from build123d import *

# Parameters (mm, degrees)
F0_W     = 20
F0_H     = 20
F1_DEPTH = 30
F3_D     = 8
F3_DEPTH = 50
F3_TIP   = 2.4034424761
F4_R     = 5
F5_W     = 20
F5_H     = 13
F6_DEPTH = 0.5


# Not quite as in the source:
# - a feature names something its author has since deleted; it is built from what else it names


with BuildPart() as f1:
    # F0 (on Right) → F1 (new body)
    with BuildSketch(Plane.YZ):
        with Locations((-10, 10)):
            Rectangle(F0_W, F0_H)
    extrude(amount=F1_DEPTH)

    # F3
    with Locations(Plane.YZ.offset(30)):
        with Locations((-10, 18.097827211)):
            Hole(F3_D / 2, depth=F3_DEPTH)
            with Locations((0, 0, -(F3_DEPTH + F3_TIP / 2))):  # 118° drill point
                Cone(0, F3_D / 2, F3_TIP, mode=Mode.SUBTRACT)

    # F4
    f4_edges = [f1.edges().sort_by_distance(p)[0] for p in [
        (30, -3.240615, 20),
        (30, -16.759385, 20),
        (15, -20, 20),
        (15, 0, 20),
        (0, -16.759385, 20),
        (0, -3.240615, 20),
    ]]
    fillet(f4_edges, radius=F4_R)

    # F5 (on face) → F6 (cut)
    with BuildSketch(Plane(origin=(0, 0, 0), x_dir=(1, 0, 0), z_dir=(0, 0, -1))):
        with Locations((15, 9.8333333333)):
            Rectangle(F5_W, F5_H)
    extrude(amount=-F6_DEPTH, mode=Mode.SUBTRACT)


solid = f1.part
Verification items for the finished model (mm, model axes). A direction names the side the tool comes from. Give positions to 0.01 mm unless a question says otherwise; leave off trailing zeros. Order: outer loops, then holes, each group sorted by start corner. A loop starts at its lowest first (then second) coordinate and runs counter-clockwise, first axis right, second up. Notation, with made-up numbers: M 60,6.5 L 66,6.5 A29 ccw 66,35.5 Z; hole C 50.25,49 d9. An arc over 180 degrees is marked long. Answer as a JSON object with one key per item and string values. Group by question number.
1) Mould release check, pull along Y, two halves, no side actions. Record for faces 1 (the face through (30, -10, 8)), 2 (the face through (14.8, -9.9, 14.1)), 3 (the face through (15, -2, 19)): released by +Y, released by -Y, zero draft, split by the parting line, or undercut.
2) Cross-section at C-C (x = 10.5). Enter the section's corners in (y, z).
3) Depth check by flat-ended pin: pin 1 Ø1.5 at (y, z) = (-15, 16.5) entering from -X; pin 2 Ø4 at (x, y) = (18.5, -9.5) entering from -Z. Enter the tip coordinate at first touch or a pass-through.
4) Cross-section at A-A (y = -10). Enter the section's corners in (x, z).
5) Access from +Z, -Z, +X, -X, +Y, -Y to the whole of each face (thin tool, end or side, straight path). Record for faces 4 (the face through (15, -10, 0.5)), 5 (the face through (1, -16, 18)).
6) Cross-section at B-B (z = 16). Enter the section's corners in (x, y), then the cut area to 3 significant figures.
7) Scan lines: line 1 along X through (y, z) = (-2, 15.25); line 2 along Z through (x, y) = (22, -10); line 3 along Y through (x, z) = (3.5, 14.75). Record each from-to range of solid material in increasing order. Write a range as [from, to].
8) Cross-section at D-D (y = -17). Enter the section's corners in (x, z), then the cut area to 3 significant figures.
Result sheet:
{
 "1": {"face 1": "zero draft", "face 2": "undercut", "face 3": "released by +Y"},
 "2": {"outline": "M -20,0 L -16.33,0 L -16.33,0.5 L -3.33,0.5 L -3.33,0 L 0,0 L 0,15 A5 ccw -5,20 L -6.48,20 A4 cw long -13.52,20 L -15,20 A5 ccw -20,15 Z"},
 "3": {"pin 1": "stops at x = 0.06", "pin 2": "stops at z = 0.5"},
 "4": {"outline": "M 0,0 L 5,0 L 5,0.5 L 25,0.5 L 25,0 L 30,0 L 30,14.1 L 0,14.1 Z"},
 "5": {"face 4": "-Z", "face 5": "+Z, -X, +Y, -Y"},
 "6": {"outline": "M 0.1,-19.9 L 29.9,-19.9 L 29.9,-13.41 L 0.1,-13.41 Z; M 0.1,-6.59 L 29.9,-6.59 L 29.9,-0.1 L 0.1,-0.1 Z", "area": "387 mm2"},
 "7": {"line 1": "x = [0.01, 29.99]", "line 2": "z = [0.5, 14.1]", "line 3": "y = [-20, -12.19], [-7.81, 0]"},
 "8": {"outline": "M 0,0 L 30,0 L 30,15 A5 ccw 27,19.58 L 3,19.58 A5 ccw 0,15 Z", "area": "580 mm2"}
}
